from build123d import *

# Parameters (mm, degrees)
F0_W            = 20
F0_H            = 24.5
F1_DEPTH        = 2
F2_W            = 20
F2_H            = 3
F3_DEPTH        = 70
F4_W            = 71
F4_H            = 4
F5_DEPTH        = 3
F6_W            = 71
F6_H            = 4
F7_DEPTH        = 3
F8_W            = 2
F8_H            = 4
F9_DEPTH        = 18.5
F10_SIZE        = 5
F11_W           = 10
F11_H           = 10
F12_DEPTH       = 3
F14_D           = 5
F14_CSINK_D     = 7
F14_CSINK_ANGLE = 90


with BuildPart() as f1:
    # F0 (on Top) → F1 (new body)
    with BuildSketch(Plane.XY):
        Rectangle(F0_W, F0_H)
    extrude(amount=F1_DEPTH)

    # F2 (on face) → F3 (join)
    with BuildSketch(Plane.XY.offset(2)):
        with Locations((0, 10.75)):
            Rectangle(F2_W, F2_H)
        with Locations((0, -10.75)):
            Rectangle(F2_W, F2_H)
    extrude(amount=F3_DEPTH)

    # F4 (on face) → F5 (join, through all)
    with BuildSketch(Plane.XZ.offset(12.25)):
        with Locations((35.5, 70)):
            Rectangle(F4_W, F4_H)
        with Locations((-35.5, 70)):
            Rectangle(F4_W, F4_H)
    extrude(amount=-F5_DEPTH)

    # F6 (on face) → F7 (join, through all)
    with BuildSketch(Plane.XZ.offset(-9.25)):
        with Locations((-35.5, 70)):
            Rectangle(F6_W, F6_H)
        with Locations((35.5, 70)):
            Rectangle(F6_W, F6_H)
    extrude(amount=-F7_DEPTH)

    # F8 (on face) → F9 (join, through all)
    with BuildSketch(Plane.XZ.offset(-9.25)):
        with Locations((-70, 70)):
            Rectangle(F8_W, F8_H)
        with Locations((70, 70)):
            Rectangle(F8_W, F8_H)
    extrude(amount=F9_DEPTH)

    # F10
    f10_edges = [f1.edges().sort_by_distance(p)[0] for p in [
        (10, 10.75, 68),
        (10, -10.75, 68),
        (-10, 10.75, 68),
        (-10, -10.75, 68),
    ]]
    chamfer(f10_edges, length=F10_SIZE)

    # F11 (on face) → F12 (join, through all)
    with BuildSketch(Plane(origin=(0, 12.25, 0), x_dir=(-1, 0, 0), z_dir=(0, 1, 0))):
        with Locations((-56, 63)):
            Rectangle(F11_W, F11_H)
        with Locations((56, 63)):
            Rectangle(F11_W, F11_H)
    extrude(amount=-F12_DEPTH)

    # F14 (through all)
    with Locations(Plane.XZ.offset(-9.25)):
        with Locations((56, 63), (-56, 63)):
            CounterSinkHole(F14_D / 2, F14_CSINK_D / 2, counter_sink_angle=F14_CSINK_ANGLE)


solid = f1.part
CAD build for the part. Positions are in the model's coordinates, mm. A direction names the side the tool comes from. Round coordinates to 2 decimals unless told otherwise and drop trailing zeros. Order: outer loops, then holes, each group sorted by start corner. A loop starts at its lowest first (then second) coordinate and runs counter-clockwise, first axis right, second up. Notation, with made-up numbers: (-1, 11) - (43, 11) arc R18 cw to (43, 40) - close; hole circle Ø4 at (-35, -19). An arc over 180 degrees is marked (long way). Return JSON: item names as keys, results as strings.
(1) Tool access for faces 1 (the face through (61, 11, 63)), 2 (the face through (-69, 0, 70)), 3 (the face through (13, 11, 66)): list every direction of +Z, -Z, +X, -X, +Y, -Y with a clear straight run to the whole face (end or side of a thin tool).
Answer key:
{"face 1": "-Z, +X, +Y, -Y", "face 2": "+Z, -Z", "face 3": "-Z, +Y, -Y"}
(2) Pull direction Z, two halves, no side cores. Call faces 4 (the face through (0, 10, 72)), 5 (the face through (53.69, 11.26, 62.04)), 6 (the face through (-12, 11, 65)): +Z half, -Z half, draft (parallel to the pull), parting line (faces both ways), or undercut.
Answer key:
{"face 4": "+Z half", "face 5": "undercut", "face 6": "-Z half"}
(3) Cut at D-D (x = 56). Give the cut face in (y, z), then the cut area to 3 significant figures.
Answer key:
{"outline": "(-12.25, 68) - (-9.25, 68) - (-9.25, 72) - (-12.25, 72) - close; (9.25, 58) - (12.25, 58) - (12.25, 60.5) - (10.25, 60.5) - (9.25, 59.5) - close; (9.25, 66.5) - (10.25, 65.5) - (12.25, 65.5) - (12.25, 72) - (9.25, 72) - close", "area": "38.0 mm^2"}
(4) Cut at C-C (y = 6). Give the cut face in (x, z), then the cut area to 3 significant figures.
Answer key:
{"outline": "(-71, 68) - (-69, 68) - (-69, 72) - (-71, 72) - close; (-10, 0) - (10, 0) - (10, 2) - (-10, 2) - close; (69, 68) - (71, 68) - (71, 72) - (69, 72) - close", "area": "56.0 mm^2"}
(5) Wall check: probe 1 along X at (y, z) = (11.8, 63); probe 2 along Y at (x, z) = (-5.5, 6); probe 3 along Z at (x, y) = (56, 11.35). Give the ranges that are in metal, low to high. Write a range as from..to.
Answer key:
{"probe 1": "x = -61..-58.5, -53.5..-51, -10..10, 51..53.5, 58.5..61", "probe 2": "y = -12.25..-9.25, 9.25..12.25", "probe 3": "z = 58..60.5, 65.5..72"}
(6) Pin check, flat tips, straight feed: pin 1 Ø3.5 at (x, y) = (-40, 10.5) entering from -Z; pin 2 Ø2.5 at (y, z) = (11, 63) entering from +X; pin 3 Ø6 at (x, y) = (-51.5, 5) entering from +Z; pin 4 Ø1.5 at (x, y) = (-57, 10.5) entering from -Z. Stop position of each tip, or through.
Answer key:
{"pin 1": "stops at z = 68", "pin 2": "stops at x = 61", "pin 3": "passes through", "pin 4": "stops at z = 58"}
(7) Cut at A-A (x = -12.5). Give the cut face in (y, z), then the cut area to 3 significant figures.
Answer key:
{"outline": "(-12.25, 65.5) - (-9.25, 65.5) - (-9.25, 72) - (-12.25, 72) - close; (9.25, 65.5) - (12.25, 65.5) - (12.25, 72) - (9.25, 72) - close", "area": "39.0 mm^2"}
(8) Cut at B-B (z = 52.5). Give the cut face in (x, y).
Answer key:
{"outline": "(-10, -12.25) - (10, -12.25) - (10, -9.25) - (-10, -9.25) - close; (-10, 9.25) - (10, 9.25) - (10, 12.25) - (-10, 12.25) - close"}
